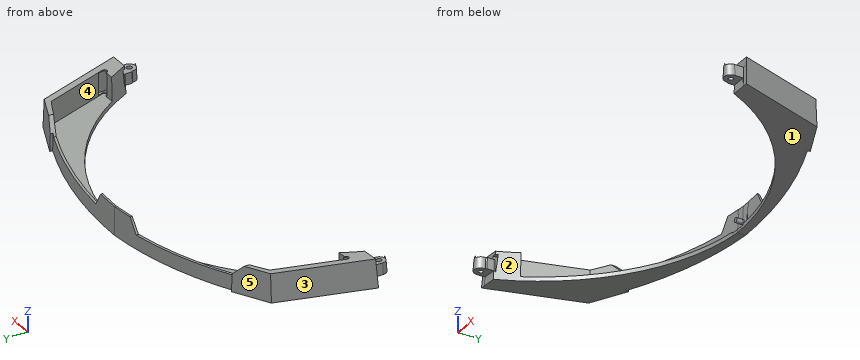
from build123d import *

# Parameters (mm, degrees)
ESQUISSE1_R             = 0.75
BOSS_EXTRU_1_DEPTH      = 10
BOSS_EXTRU_1_DRAFT      = 2
ESQUISSE2_W             = 13.85789223
ESQUISSE2_H             = 8.60111757
ENL_V_MAT_EXTRU_1_DEPTH = 13
ESQUISSE5_W             = 12.990785821
ESQUISSE5_H             = 5.57811828
ENL_V_MAT_EXTRU_3_DEPTH = 13
ENL_V_MAT_EXTRU_4_DEPTH = 18.5
ESQUISSE8_W             = 3.624703647
ESQUISSE8_H             = 8.1
ENL_V_MAT_EXTRU_7_DEPTH = 9
ENL_V_MAT_EXTRU_7_DRAFT = -6
ENL_V_MAT_EXTRU_8_DEPTH = 6.5
ENL_V_MAT_EXTRU_6_DEPTH = 24
ESQUISSE12_R            = 1.011324244
ENL_V_MAT_EXTRU_9_DEPTH = 6
ESQUISSE17_R            = 0.825
BOSS_EXTRU_2_DEPTH      = 2


# Read off the part's stored shape, not the designer's step: Symétrie2
with BuildPart() as part:
    # Esquisse1 → Boss.-Extru.1 (with draft: the straight prism first)
    with BuildSketch(Plane.XY):
        with BuildLine():
            Line((77.8887043, -44.926917936), (67.208968034, -12.647772451))
            Line((67.208968034, -12.647772451), (53.475934981, -6.614216024))
            Line((53.475934981, -6.614216024), (53.395110551, -7.610944377))
            ThreePointArc((53.395110551, -7.610944377), (27.216820071, 0.300239401), (0, 2.971274119))
            Line((0, 2.971274119), (0, 0))
            ThreePointArc((0, 0), (41.918820025, -12.179976378), (70.783627584, -44.926917936))
            Line((70.783627584, -44.926917936), (70.783627584, -47.429888392))
            Line((70.783627584, -47.429888392), (71.170117615, -47.747103549))
            ThreePointArc((71.170117615, -47.747103549), (73.573677122, -50.425298655), (76.163642587, -47.926917936))
            Line((76.163642587, -47.926917936), (76.163642587, -44.926917936))
            Line((76.163642587, -44.926917936), (77.8887043, -44.926917936))
        make_face()
        with Locations((73.663642587, -47.926917936)):
            Circle(ESQUISSE1_R, mode=Mode.SUBTRACT)
    extrude(amount=BOSS_EXTRU_1_DEPTH)
    # Boss.-Extru.1: the draft: its side faces are tilted about the plane it starts from
    boss_extru_1_sides = [part.faces().sort_by_distance(p)[0] for p in [
        (72.548836167, -28.787345194, 5),
        (60.342451508, -9.630994237, 5),
        (53.435522766, -7.1125802, 5),
        (27.216820071, 0.300239401, 5),
        (0, 1.48563706, 5),
        (41.918820025, -12.179976378, 5),
        (70.783627584, -46.178403164, 5),
        (70.9768726, -47.588495971, 5),
        (73.573677122, -50.425298655, 5),
        (76.163642587, -46.426917936, 5),
        (77.026173444, -44.926917936, 5),
        (72.913642587, -47.926917936, 5),
    ]]
    draft(boss_extru_1_sides, Plane.XY, BOSS_EXTRU_1_DRAFT)

    # Esquisse2 → Enlèv. mat.-Extru.1 (cut)
    with BuildSketch(Plane(origin=(0, 0, -10), x_dir=(-1, 0, 0), z_dir=(0, 0, -1))):
        with Locations((-70.959758185, -49.227476721)):
            Rectangle(ESQUISSE2_W, ESQUISSE2_H)
    extrude(amount=-ENL_V_MAT_EXTRU_1_DEPTH, mode=Mode.SUBTRACT)

    # Esquisse5 → Enlèv. mat.-Extru.3 (cut)
    with BuildSketch(Plane.XY.offset(20)):
        with Locations((70.909949533, -47.366769381)):
            Rectangle(ESQUISSE5_W, ESQUISSE5_H)
    extrude(amount=-ENL_V_MAT_EXTRU_3_DEPTH, mode=Mode.SUBTRACT)

    # Esquisse6 → Enlèv. mat.-Extru.4 (cut)
    with BuildSketch(Plane.XY.offset(20)):
        with BuildLine():
            Line((64.669985027, -14.044516655), (72.45607407, -37.577710241))
            ThreePointArc((72.45607407, -37.577710241), (71.45607407, -38.577710241), (70.45607407, -37.577710241))
            Line((70.45607407, -37.577710241), (2.849207695, -37.577710241))
            Line((2.849207695, -37.577710241), (2.849207695, 1.892851629))
            ThreePointArc((2.849207695, 1.892851629), (34.687321508, -2.477202631), (64.669985027, -14.044516655))
        make_face()
    extrude(amount=-ENL_V_MAT_EXTRU_4_DEPTH, mode=Mode.SUBTRACT)


with BuildPart() as enl_v_mat_extru_7_tool:
    # Esquisse8 → Enlèv. mat.-Extru.7 (with draft: the straight prism first)
    with BuildSketch(Plane(origin=(0, -35.577710241, 0), x_dir=(1, 0, 0), z_dir=(0, 1, 0))):
        with Locations((71.507795019, -5.75)):
            Rectangle(ESQUISSE8_W, ESQUISSE8_H)
    extrude(amount=-ENL_V_MAT_EXTRU_7_DEPTH)
    # Enlèv. mat.-Extru.7: the draft: its side faces are tilted about the plane it starts from
    enl_v_mat_extru_7_sides = [enl_v_mat_extru_7_tool.faces().sort_by_distance(p)[0] for p in [
        (69.695443195, -40.077710241, 5.75),
        (71.507795019, -40.077710241, 9.8),
        (73.320146842, -40.077710241, 5.75),
        (71.507795019, -40.077710241, 1.7),
    ]]
    draft(enl_v_mat_extru_7_sides, Plane(origin=(0, -35.577710241, 0), x_dir=(1, 0, 0), z_dir=(0, 1, 0)), ENL_V_MAT_EXTRU_7_DRAFT)


with BuildPart() as part_1:
    add(part.part)

    # Enlèv. mat.-Extru.7: cut by enl_v_mat_extru_7_tool
    add(enl_v_mat_extru_7_tool.part, mode=Mode.SUBTRACT)

    # Esquisse9 → Enlèv. mat.-Extru.8 (cut)
    with BuildSketch(Plane(origin=(0, -4.896564999, 0.170991818), x_dir=(0.9999999998537095, -5.969561417335715e-07, -1.7094587273474584e-05), z_dir=(0, 0.9993908270190958, -0.03489949670250105))):
        with BuildLine():
            Line((3.349657801, -1.114368939), (0.03533908, -1.114368939))
            Line((0.03533908, -1.114368939), (0.119413388, -3.518714663))
            ThreePointArc((0.119413388, -3.518714663), (1.002393791, -4.338878244), (0.178858385, -5.218714663))
            Line((0.178858385, -5.218714663), (0.349657801, -10.103213324))
            Line((0.349657801, -10.103213324), (3.349657801, -10.111959186))
            Line((3.349657801, -10.111959186), (3.349657801, -1.114368939))
        make_face()
    extrude(amount=ENL_V_MAT_EXTRU_8_DEPTH, mode=Mode.SUBTRACT)

    # Esquisse7 → Enlèv. mat.-Extru.6 (cut)
    with BuildSketch(Plane(origin=(0, 5.097343272, -0.178003149), x_dir=(0.9999999998537095, -5.969561417335715e-07, -1.7094587273474584e-05), z_dir=(0, 0.9993908270190958, -0.03489949670250105))):
        Polygon((12, -5.000000781), (9, -10.085416779), (58.325804645, -10.085411957), (52.617108891, -5.000000781), align=None)
    extrude(amount=-ENL_V_MAT_EXTRU_6_DEPTH, mode=Mode.SUBTRACT)

    # Symétrie2: part across plane


with BuildPart() as part_2:
    add(part_1.part)
    add(part_1.part.mirror(Plane(origin=(0, 0, 0), x_dir=(0.034899496702501046, 0, 0.9993908270190957), z_dir=(-0.9993908270190958, 0, 0.034899496702501046))))

    # Esquisse12 → Enlèv. mat.-Extru.9 (cut)
    with BuildSketch(Plane(origin=(0, -4.896564999, 0.170991818), x_dir=(0.9999999998537095, -5.969561417335715e-07, -1.7094587273474584e-05), z_dir=(0, 0.9993908270190958, -0.03489949670250105))):
        with Locations((0.159665326, -4.247929052)):
            Circle(ESQUISSE12_R)
    extrude(amount=ENL_V_MAT_EXTRU_9_DEPTH, mode=Mode.SUBTRACT)

    # Esquisse17 → Boss.-Extru.2 (add)
    with BuildSketch(Plane(origin=(0, 1.099779964, -0.038405163), x_dir=(-1, 0, 0), z_dir=(0, -0.9993908270190958, 0.03489949670250106))):
        with Locations(Location((-0.146292507, -4.268691639, 0), (0, 0, 9.44628294))):
            Circle(ESQUISSE17_R)
    extrude(amount=BOSS_EXTRU_2_DEPTH)


solid = part_2.part
The listing builds one solid part. Answer for the finished solid, in the listing's coordinates (mm). Face numbers are marked on the shaded views. A direction names the side the tool comes from. Give positions to 0.01 mm unless a question says otherwise; leave off trailing zeros. Answer as a JSON object with one key per item and string values.
1. For the marked faces 4 and 5, determine the directions among +Z, -Z, +X, -X, +Y, -Y from which every point of the face is accessible in a straight line to the end or side of a thin tool.
Determined:
{"face 4": "+Z", "face 5": "+Z, -X, +Y"}
2. For a pull along X with two mould halves and no side action, classify the marked faces 1, 2 and 3 as pulls with the +X half, pulls with the -X half, needs draft (parallel to the pull), parting line crosses it, or undercut.
Determined:
{"face 1": "needs draft", "face 2": "undercut", "face 3": "pulls with the -X half"}
3. Find the intervals of material crossed by L1, parallel to X at y = -38, z = 7.5 (3 decimals); L2, parallel to X at y = -21, z = 1.25; L3, parallel to Y at x = -3.5, z = 3, in increasing order. Write a range as [from, to].
Determined:
{"L1": "[-75.175, -72.72], [-69.596, -66.844], [67.395, 69.95], [73.066, 75.321]", "L2": "[53.4, 69.93]", "L3": "[1.87, 2.83]"}
4. Flat-ended cylindrical pins translate along their axes: pin 1 Ø5 at (y, z) = (-38.5, 13.5) entering from -X; pin 2 Ø2.5 at (x, z) = (-72, 11.5) entering from -Y; pin 3 Ø6 at (x, z) = (19.5, 2) entering from +Y. Find the tip coordinate at first contact, or state that the pin passes through.
Determined:
{"pin 1": "x = -75.57", "pin 2": "y = -50.23", "pin 3": "y = 1.94"}
